Read the model definition and answer for the solid it produces. Units are mm, in the model's axes. A direction names the side the tool comes from. Coordinates: 2 decimals unless noted, no trailing zeros. Write each loop counter-clockwise with the first axis right and the second up, starting at its lowest first coordinate (ties: lowest second). Pieces come first, ordered by that corner, then holes. Notation, with made-up numbers: M 48.5,65.25 L 101.5,65.25 A21 cw 101.5,79.25 Z; hole C -7.5,24 d4. An arc over 180 degrees is marked long. Use a Markdown table: item, result. Add a question column.
Autodesk Inventor part; units mm, degrees
ref_plane "YZ Plane" through (0, 0, 0) normal (1, 0, 0) x (0, 1, 0)
ref_plane "XZ Plane" through (0, 0, 0) normal (0, 1, 0) x (-1, 0, 0)
ref_plane "XY Plane" through (0, 0, 0) normal (0, 0, 1) x (1, 0, 0)
sketch "Sketch1" plane through (0, 0, 0) normal (0, 1, 0) x (-1, 0, 0)
  line L0 (-7.3056, 10.788) -> (-92.3056, 10.788)
  line L1 (-92.3056, 10.788) -> (-92.3056, -74.212)
  line L2 (-92.3056, -74.212) -> (-7.3056, -74.212)
  line L3 (-7.3056, -74.212) -> (-7.3056, 10.788)
  line L4 (-18.8056, -21.212) -> (-59.8056, -21.212)
  line L5 (-59.8056, -21.212) -> (-59.8056, -42.212)
  line L6 (-59.8056, -42.212) -> (-18.8056, -42.212)
  line L7 (-18.8056, -42.212) -> (-18.8056, -21.212)
  circle A0 centre (-14.3056, -26.712) radius 1.3
  circle A1 centre (-14.3056, -36.712) radius 1.3
  circle A2 centre (-64.3056, -26.712) radius 1.3
  circle A3 centre (-64.3056, -36.712) radius 1.3
  circle A4 centre (-75.3056, -39.212) radius 1.3
  circle A5 centre (-85.3056, -39.212) radius 1.3
  circle A6 centre (-75.3056, -24.212) radius 1.3
  circle A7 centre (-85.3052, -24.1286) radius 1.3
  point P0 (0, 0)
  dimension "d0" = 85
  dimension "d1" = 85
  dimension "d2" = 41
  dimension "d3" = 21
  dimension "d4" = 32
  dimension "d5" = 11.5
  dimension "d6" = 2.6
  dimension "d7" = 2.6
  dimension "d8" = 10
  dimension "d9" = 5.5
  dimension "d10" = 5.5
  dimension "d11" = 2.6
  dimension "d12" = 2.6
  dimension "d13" = 10
  dimension "d14" = 5.5
  dimension "d15" = 50
  dimension "d16" = 50
  dimension "d17" = 4.5
  dimension "d31" = 2.6
  dimension "d32" = 2.6
  dimension "d33" = 10
  dimension "d34" = 2.6
  dimension "d35" = 2.6
  dimension "d36" = 10
  dimension "d37" = 15
  dimension "d38" = 35
  dimension "d39" = 17
  dimension "d40" = 17
extrude "Extrusion1" add sketch "Sketch1" along normal blind 2.8 contours L3 L2 L1 L0 | A4 | A5 | A6 | A7
sketch "Sketch2" plane through (0, 2.8, 0) normal (0, 1, 0) x (1, 0, 0)
  line L0 (92.3056, -10.788) -> (92.3056, 74.212)
  line L1 (92.3056, 74.212) -> (7.3056, 74.212)
  line L2 (7.3056, -10.788) -> (92.3056, -10.788)
  point P0 (0, 0)
extrude "Extrusion2" [suppressed]
sketch "Sketch3" plane through (0, 2.8, 0) normal (0, 1, 0) x (1, 0, 0)
  line L0 (7.3056, -10.788) -> (92.3056, -10.788)
  line L1 (92.3056, 74.212) -> (7.3056, 74.212)
  line L2 (92.3056, -10.788) -> (69.6056, -10.788)
  line L3 (69.6056, -10.788) -> (69.6056, 74.212)
  line L4 (69.6056, 74.212) -> (92.3056, 74.212)
  line L5 (92.3056, 74.212) -> (92.3056, -10.788)
  circle A0 centre (64.3056, 36.712) radius 1.3
  circle A1 centre (75.3056, 24.212) radius 1
  circle A2 centre (75.3056, 24.212) radius 1
  circle A3 centre (75.3056, 39.212) radius 1
  circle A4 centre (75.3056, 39.212) radius 1
  circle A5 centre (85.3056, 39.212) radius 1
  circle A6 centre (85.3056, 39.212) radius 1
  circle A7 centre (85.3056, 24.212) radius 1
  circle A8 centre (85.3056, 24.212) radius 1
  circle A9 centre (84.8056, 66.712) radius 0.95
  circle A10 centre (84.8056, 66.712) radius 1
  circle A11 centre (84.8056, -3.288) radius 0.95
  circle A12 centre (84.8056, -3.288) radius 1
  point P0 (0, 0)
  dimension "d55" = 4
  dimension "d56" = 2
  dimension "d57" = 2
extrude "Extrusion3" add sketch "Sketch3" along normal blind 27 contours L3 L1 L5 L0
sketch "Sketch4" plane through (92.3056, 0, 10.788) normal (1, 0, 0) x (0, 0, -1)
  line L0 (85, 2.8) -> (0, 2.8)
  line L1 (2.5, 27.3) -> (82.5, 27.3)
  line L2 (82.5, 27.3) -> (82.5, 2.8)
  line L3 (82.5, 2.8) -> (2.5, 2.8)
  line L4 (2.5, 2.8) -> (2.5, 27.3)
  line L5 (0, 0) -> (0, 29.8)
  line L6 (85, 0) -> (85, 29.8)
  line L7 (0, 0) -> (85, 0)
  line L8 (0, 29.8) -> (85, 29.8)
  point P0 (10.788, 0)
  point P1 (2.5, 2.8)
  dimension "d60" = 2.5
  dimension "d61" = 2.5
  dimension "d62" = 2.8
  dimension "d63" = 2.5
extrude "Extrusion4" cut sketch "Sketch4" against normal blind 21 contours L0 L4 L1 L2
sketch "Sketch5" plane through (0, 0, 0) normal (0, -1, 0) x (1, 0, 0)
  circle A0 centre (26.7535, -8.6599) radius 1.3
  circle A1 centre (72.8576, -8.66) radius 1.3
  circle A2 centre (26.7536, -54.764) radius 1.3
  circle A3 centre (72.8576, -54.764) radius 1.3
  line L0 (7.3056, 10.788) -> (92.3056, 10.788)
  line L1 (92.3056, 10.788) -> (92.3056, -74.212)
  line L2 (7.3056, -74.212) -> (7.3056, 10.788)
  line L3 (92.3056, -74.212) -> (7.3056, -74.212)
  point P0 (0, 0)
  point P1 (49.2547, -32.4518)
  point P2 (49.2547, -32.4518)
  dimension "d66" = 2.6
  dimension "d67" = 2.6
  dimension "d68" = 2.6
  dimension "d69" = 2.6
  dimension "d70" = 46.1041
  dimension "d71" = 46.1041
  dimension "d72" = 46.1041
  dimension "d73" = 46.1041
  dimension "d74" = 19.448
  dimension "d75" = 19.448
  dimension "d76" = 19.448
  dimension "d77" = 19.448
extrude "Extrusion5" cut sketch "Sketch5" against normal blind 100 contours A0 | A1 | A2 | A3
sketch "Sketch6" plane through (0, 29.8, 0) normal (0, 1, 0) x (1, 0, 0)
  point P0 (0, 0)
sketch "Sketch7" plane through (0, 29.8, 0) normal (0, 1, 0) x (1, 0, 0)
  circle A0 centre (75.3056, 39.212) radius 1
  circle A1 centre (75.3056, 39.212) radius 1.3
  circle A2 centre (85.3056, 39.212) radius 1
  circle A3 centre (85.3056, 39.212) radius 1.3
  circle A4 centre (75.3056, 24.212) radius 1
  circle A5 centre (75.3056, 24.212) radius 1.3
  circle A6 centre (85.3056, 24.212) radius 1
  circle A7 centre (85.3056, 24.212) radius 1.3
  point P0 (0, 0)
  dimension "d80" = 2.6
  dimension "d81" = 2.6
  dimension "d82" = 2.6
  dimension "d83" = 2.6
extrude "Extrusion6" cut sketch "Sketch7" against normal blind 10 contours A0 | A1 | A2 | A3 | A4 | A5 | A6 | A7
properties part number "LowerHead"
Item 1: Determine the mould class of faces 1 (the flat face through (71.306, 15, -31)), 2 (the cylindrical face through (84.01, 28.53, -67.32)), 3 (the flat face through (7.306, 1, -32)) for opening direction X: pulls with the +X half, pulls with the -X half, needs draft (parallel to the pull), parting line crosses it, or undercut.
Item 2: Find section C-C on z = -1.5. Give the vertices of the cut face in (x, y).
Item 3: Consider probe 1 along Z at (x, y) = (72, 18); probe 2 along Y at (x, z) = (84, -36.5); probe 3 along Y at (x, z) = (59.5, -12.5). Determine where each line is inside the solid, lowest interval first.
Item 4: Find section A-A on x = 45. Give the vertices of the cut face in (y, z).
Item 5: For faces 4 (the flat face through (18.806, 1, -32)), 5 (the cylindrical face through (83.807, 28.533, 3.332)), 6 (the flat face through (69.606, 16, -31)), determine the directions among +Z, -Z, +X, -X, +Y, -Y from which every point of the face is accessible in a straight line to the end or side of a thin tool.
Item 6: Find section B-B on y = 21. Give the vertices of the cut face in (x, z), then the cut area to 4 significant figures.
Item 7: Each of these flat-tipped pins is pushed along its axis until it touches: pin 1 (2 mm diameter, centred on y = 8.5, z = -42, fed in from +X); pin 2 (1 mm diameter, centred on y = 7.5, z = -42, fed in from -X); pin 3 (12 mm diameter, centred on x = 61, z = -55.5, fed in from +Y); pin 4 (1.6 mm diameter, centred on x = 72.86, z = -54.76, fed in from +Y). Where does it stop, or does it pass through?
Geometry says:
| question | item | result |
|---|---|---|
| 1 | face 1 | pulls with the +X half |
| 1 | face 2 | undercut |
| 1 | face 3 | pulls with the -X half |
| 2 | outline | M 7.31,0 L 92.31,0 L 92.31,2.8 L 71.31,2.8 L 71.31,27.3 L 92.31,27.3 L 92.31,29.8 L 69.61,29.8 L 69.61,2.8 L 7.31,2.8 Z |
| 3 | probe 1 | z = -74.21 to -71.71, 8.29 to 10.79 |
| 3 | probe 2 | y = 0 to 2.8, 27.3 to 29.8 |
| 3 | probe 3 | y = 0 to 2.8 |
| 4 | outline | M 0,-74.21 L 2.8,-74.21 L 2.8,-42.21 L 0,-42.21 Z; M 0,-21.21 L 2.8,-21.21 L 2.8,10.79 L 0,10.79 Z |
| 5 | face 4 | +Y, -Y |
| 5 | face 5 | +Y |
| 5 | face 6 | +Z, -Z, -X, +Y |
| 6 | outline | M 69.61,-74.21 L 92.31,-74.21 L 92.31,-71.71 L 71.31,-71.71 L 71.31,8.29 L 92.31,8.29 L 92.31,10.79 L 69.61,10.79 Z |
| 6 | area | 249.5 mm2 |
| 7 | pin 1 | stops at x = 71.31 |
| 7 | pin 2 | stops at x = 69.61 |
| 7 | pin 3 | stops at y = 2.8 |
| 7 | pin 4 | passes through |
